```python
from build123d import *

# Parameters (mm, degrees)
SKETCH1_W           = 457.2
SKETCH1_H           = 203.2
BOSS_EXTRUDE1_DEPTH = 12.7
CUT_EXTRUDE1_START  = -26.4
SKETCH2_R           = 12.7
CUT_EXTRUDE1_DEPTH  = 27.4


with BuildPart() as part:
    # Sketch1 → Boss-Extrude1 (new body, symmetric)
    with BuildSketch(Plane(origin=(0, 0, 0), x_dir=(0, 0, -1), z_dir=(1, 0, 0))):
        with Locations((228.6, 101.6)):
            Rectangle(SKETCH1_W, SKETCH1_H)
    extrude(amount=BOSS_EXTRUDE1_DEPTH, both=True)

    # Sketch2 → Cut-Extrude1 (cut)
    with BuildSketch(Plane.ZY.offset(12.7).offset(CUT_EXTRUDE1_START)):
        with Locations((-431.8, 101.6)):
            Circle(SKETCH2_R)
    cut_extrude1 = extrude(amount=CUT_EXTRUDE1_DEPTH, mode=Mode.SUBTRACT)

    # Mirror3: Cut-Extrude1 across plane
    add(cut_extrude1.mirror(Plane.XY.offset(-228.6)), mode=Mode.SUBTRACT)


solid = part.part
```
For this review, take the finished solid that the model builds, in its own axes (mm). Coordinates: 2 decimals unless noted, no trailing zeros. Loops run counter-clockwise (first coordinate to the right, second up) from the corner with the lowest first, then second, coordinate; pieces in that order, holes last. Notation, with made-up numbers: (38, 27) -> (44, 27) arc R26 cw to (44, 61) -> close; hole circle Ø10 at (29.5, -16). An arc over 180 degrees is marked (long way). Return JSON: item names as keys, results as strings. Group by question number.
(1) Consider section B-B, the plane y = 101.6. Give the boundary of the cut face in (x, z), plus the area to 3 significant figures.
(2) Mouldability with a two-part tool opening along Y and no side actions: class faces 1 (the flat face through (0, 203.2, -225)), 2 (the flat face through (0, 0, -225)), 3 (the cylindrical face through (0.178, 114.192, -433.453)), 4 (the flat face through (0, 100, -457.2)) as pulls with the +Y half, pulls with the -Y half, needs draft (parallel to the pull), parting line crosses it, or undercut.
(3) For pin 1 Ø5 at (x, y) = (3, 57.5) entering from +Z, flat-tipped, find the tip position at first contact; note if it passes through.
(4) To check wall thickness, follow L1, parallel to Z at x = -10, y = 101.5; L2, parallel to Y at x = 5.75, z = -431.8; L3, parallel to Z at x = -3, y = 96. State the ranges of each line that lie inside material, in increasing order.
(5) Consider section A-A, the plane z = -25.4. Give the boundary of the cut face in (x, y), plus the area to 3 significant figures.
Results below:
{
 "1": {"outline": "(-12.7, -457.2) -> (12.7, -457.2) -> (12.7, -444.5) -> (-12.7, -444.5) -> close; (-12.7, -419.1) -> (12.7, -419.1) -> (12.7, -38.1) -> (-12.7, -38.1) -> close; (-12.7, -12.7) -> (12.7, -12.7) -> (12.7, 0) -> (-12.7, 0) -> close", "area": "10,300 mm2"},
 "2": {"face 1": "pulls with the +Y half", "face 2": "pulls with the -Y half", "face 3": "undercut", "face 4": "needs draft"},
 "3": {"pin 1": "stops at z = 0"},
 "4": {"L1": "z = -457.2 to -444.5, -419.1 to -38.1, -12.7 to 0", "L2": "y = 0 to 88.9, 114.3 to 203.2", "L3": "z = -457.2 to -443.2, -420.4 to -36.8, -14 to 0"},
 "5": {"outline": "(-12.7, 0) -> (12.7, 0) -> (12.7, 88.9) -> (-12.7, 88.9) -> close; (-12.7, 114.3) -> (12.7, 114.3) -> (12.7, 203.2) -> (-12.7, 203.2) -> close", "area": "4,520 mm2"}
}
